Part model, mm, in its own coordinate system. Give positions to 0.01 mm unless a question says otherwise; leave off trailing zeros. Write each loop counter-clockwise with the first axis right and the second up, starting at its lowest first coordinate (ties: lowest second). Pieces come first, ordered by that corner, then holes. Notation, with made-up numbers: M -19.5,34 L -10.5,34 A25 cw -10.5,54 Z; hole C 62.5,16 d1. An arc over 180 degrees is marked long. Use a Markdown table: item, result. Add a question column.
from build123d import *

# Parameters (mm, degrees)
EXTRUDE_THIN1_DEPTH = 584.2
SKETCH3_W           = 15.24
SKETCH3_H           = 3.302
CUT_EXTRUDE1_DEPTH  = 142.12875


with BuildPart() as part:
    # Sketch2 → Extrude-Thin1 (new body)
    with BuildSketch(Plane(origin=(0, 0, 0), x_dir=(0, 0, -1), z_dir=(1, 0, 0))):
        with BuildLine():
            ThreePointArc((94.192253267, -105.09587766), (128.861474149, -57.550365391), (141.12875, 0))
            Line((141.12875, 0), (139.54125, 0))
            ThreePointArc((139.54125, 0), (127.411963754, -56.903004701), (93.132722859, -103.913696809))
            Line((93.132722859, -103.913696809), (94.192253267, -105.09587766))
        make_face()
    extrude(amount=EXTRUDE_THIN1_DEPTH)

    # Sketch3 → Cut-Extrude1 (cut, through all)
    with BuildSketch(Plane.XY):
        with Locations((7.62, -85.752696809)):
            Rectangle(SKETCH3_W, SKETCH3_H)
        with Locations((576.58, -85.752696809)):
            Rectangle(SKETCH3_W, SKETCH3_H)
    extrude(amount=-CUT_EXTRUDE1_DEPTH, mode=Mode.SUBTRACT)


solid = part.part
1. Cut at A-A (x = 434). Write the cut outline in (y, z), then the cut area to 3 significant figures.
2. Flat gauge pins, fed straight in: pin 1 (0.6 mm diameter, centred on x = 7, z = -109.5, fed in from +Y); pin 2 (3 mm diameter, centred on x = 516.5, z = -103, fed in from +Y); pin 3 (6 mm diameter, centred on x = 287, y = -91, fed in from -Z); pin 4 (3.5 mm diameter, centred on y = -86.5, z = -110.5, fed in from -X). Where does each tip first touch, or does it go through?
3. Cut at B-B (y = -23). Write the cut outline in (x, z), then the cut area to 3 significant figures.
4. Drill centre lines: probe 1 along Y at (x, z) = (259, -126); probe 2 along Z at (x, y) = (368, -57); probe 3 along Z at (x, y) = (294.5, -62). Where is each one in solid material? Low to high. Write a range as [from, to].
A:
| question | item | result |
|---|---|---|
| 1 | outline | M -105.1,-94.19 A141.13 ccw 0,-141.13 L 0,-139.54 A139.54 cw -103.91,-93.13 Z |
| 1 | area | 187 mm² |
| 2 | pin 1 | stops at y = -87.4 |
| 2 | pin 2 | stops at y = -92.47 |
| 2 | pin 3 | stops at z = -110.33 |
| 2 | pin 4 | stops at x = 0 |
| 3 | outline | M 0,-139.24 L 584.2,-139.24 L 584.2,-137.63 L 0,-137.63 Z |
| 3 | area | 940 mm² |
| 4 | probe 1 | y = [-63.57, -59.96] |
| 4 | probe 2 | z = [-129.11, -127.37] |
| 4 | probe 3 | z = [-126.78, -125.01] |
